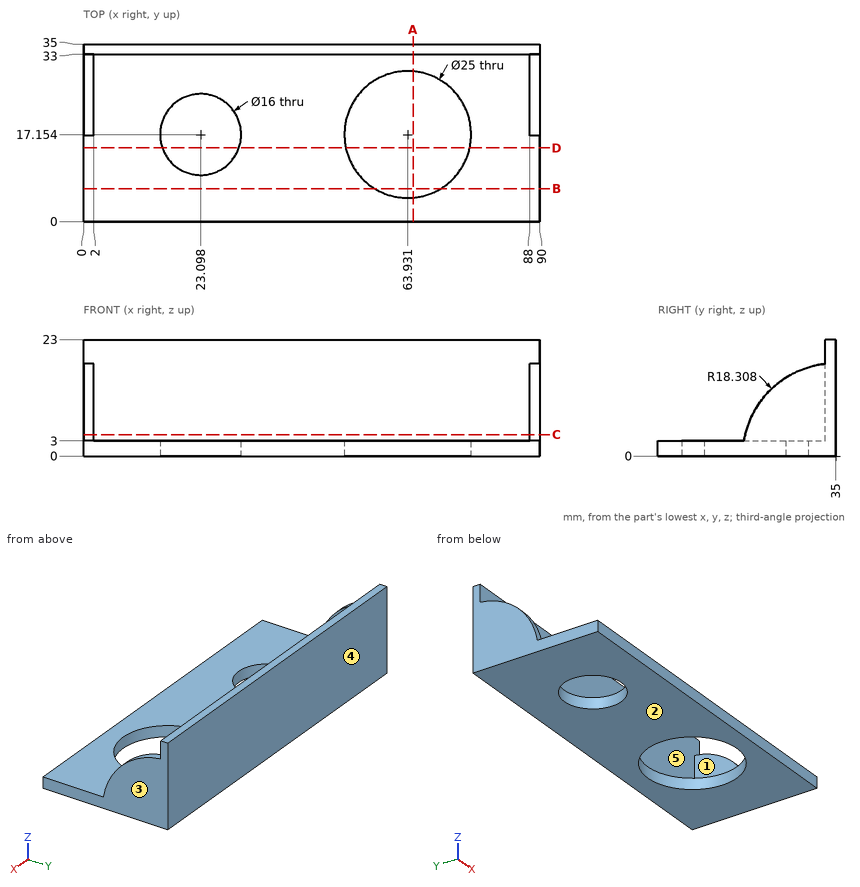
For this review, use the dimensioned drawing (mm, ordinates from the lowest corner) and the shaded views. A direction names the side the tool comes from. Round coordinates to 2 decimals unless told otherwise and drop trailing zeros. Write each loop counter-clockwise with the first axis right and the second up, starting at its lowest first coordinate (ties: lowest second). Pieces come first, ordered by that corner, then holes. Notation, with made-up numbers: M 66.5,-29.75 L 81.5,-29.75 A18 cw 81.5,2.25 Z; hole C 10.25,47.25 d5. An arc over 180 degrees is marked long. Answer as CSV lines item,"result". Start each with the question number.
Q1. Consider section D-D, the plane y = 14.5. Give the boundary of the cut face in (x, z) (1 decimal).
Q2. Tool access review of the marked faces 1 and 2: name each direction out of +Z, -Z, +X, -X, +Y, -Y from which nothing blocks a thin tool from reaching the whole face with its end or side.
Q3. Wall thickness on line 1 along X through (y, z) = (26, 6.5); line 2 along Y through (x, z) = (48, 16.75); line 3 along Z through (x, y) = (68.5, 2): over which ranges is each line inside the solid? List them lowest first.
Q4. Clearance check with flat-ended pins moving along their axes: P1, Ø5, axis at x = 49, y = 19.5, coming from the +Z side; P2, Ø2, axis at x = 61.5, z = 8, coming from the -Y side. State where each tip first meets the part, or that it passes through.
Q5. Consider section B-B, the plane y = 6.5. Give the boundary of the cut face in (x, z).
Q6. Consider section C-C, the plane z = 4.25. Give the boundary of the cut face in (x, y).
Q7. Consider section A-A, the plane x = 65. Give the boundary of the cut face in (y, z).
Q8. The part is to be moulded in two halves that separate along X. For the marked faces 3, 4 and 5, say which applies: +X half, -X half, draft (parallel to the pull), parting line (faces both ways), or undercut.
Result set:
1,outline,"M 0,0 L 15.6,0 L 15.6,3 L 0,3 Z; M 30.6,0 L 51.7,0 L 51.7,3 L 30.6,3 Z; M 76.1,0 L 90,0 L 90,3 L 76.1,3 Z"
2,face 1,"+Z, -Y"
2,face 2,"-Z, +X, -X, +Y, -Y"
3,line 1,"x = 0 to 2, 88 to 90"
3,line 2,"y = 33 to 35"
3,line 3,"z = 0 to 3"
4,P1,"stops at z = 3"
4,P2,"stops at y = 33"
5,outline,"M 0,0 L 57.39,0 L 57.39,3 L 0,3 Z; M 70.47,0 L 90,0 L 90,3 L 70.47,3 Z"
6,outline,"M 0,17.19 L 2,17.19 L 2,33 L 88,33 L 88,17.19 L 90,17.19 L 90,35 L 0,35 Z"
7,outline,"M 0,0 L 4.7,0 L 4.7,3 L 0,3 Z; M 29.61,0 L 35,0 L 35,23 L 33,23 L 33,3 L 29.61,3 Z"
8,face 3,"+X half"
8,face 4,"draft"
8,face 5,"undercut"
